```python
from build123d import *

# Parameters (mm, degrees)
BOSS_EXTRUDE1_DEPTH             = 26.5
SKETCH2_W                       = 10
SKETCH2_H                       = 15
BOSS_EXTRUDE2_DEPTH             = 21.1
BOSS_EXTRUDE2_DIRECTION_2_REACH = 46.455
SKETCH3_W                       = 13.25
SKETCH3_H                       = 38
CUT_EXTRUDE1_DEPTH              = 21.1
CUT_EXTRUDE2_DEPTH              = 46.618088518
CUT_EXTRUDE2_DEPTH_BACK         = 46.618088518
SKETCH4_R                       = 1.8
SKETCH5_R                       = 3.5
CUT_EXTRUDE3_DEPTH              = 11.1
SKETCH6_R                       = 1.9
CUT_EXTRUDE4_DEPTH              = 46.618088518
FILLET1_R                       = 5
CHAMFER1_SIZE                   = 0.25


with BuildPart() as part:
    # Sketch1 → Boss-Extrude1 (new body)
    with BuildSketch(Plane.XY):
        Polygon((0, 35), (0, 28), (2.4, 28), (2.4, -10), (7, -10), (7, 35), align=None)
    extrude(amount=BOSS_EXTRUDE1_DEPTH)

    # Sketch2 → Boss-Extrude2 (add)
    with BuildSketch(Plane.XY):
        with Locations((7.4, -2.5)):
            Rectangle(SKETCH2_W, SKETCH2_H)
    extrude(amount=-BOSS_EXTRUDE2_DEPTH)

    # Boss-Extrude2 direction 2: up to this face of the body (flat: up to its plane)
    boss_extrude2_direction_2_end = Plane(part.part.faces().sort_by_distance((4.437265416, 13.926273458, 26.5))[0])
    # Sketch2 → Boss-Extrude2 direction 2 (add, up to the picked face)
    with BuildSketch(Plane.XY, mode=Mode.PRIVATE) as boss_extrude2_direction_2_sk1:
        with Locations((7.4, -2.5)):
            Rectangle(SKETCH2_W, SKETCH2_H)
    boss_extrude2_direction_2_tool1 = split(extrude(boss_extrude2_direction_2_sk1.sketch, amount=BOSS_EXTRUDE2_DIRECTION_2_REACH, mode=Mode.PRIVATE), bisect_by=boss_extrude2_direction_2_end, keep=Keep.BOTH, mode=Mode.PRIVATE)
    add(boss_extrude2_direction_2_tool1.solids().sort_by(Axis((7.4, -2.5, 0), (0, 0, 1)))[0])

    # Sketch3 → Cut-Extrude1 (cut)
    with BuildSketch(Plane(origin=(0, 0, 0), x_dir=(0, 0, -1), z_dir=(1, 0, 0))):
        with Locations((-19.875, 9)):
            Rectangle(SKETCH3_W, SKETCH3_H)
    extrude(amount=CUT_EXTRUDE1_DEPTH, mode=Mode.SUBTRACT)

    # Sketch4 → Cut-Extrude2 (cut, two sides: drawn at the far end of the back side and taken through both)
    with BuildSketch(Plane.XY.offset(-CUT_EXTRUDE2_DEPTH_BACK)):
        with Locations((7.4, -2.5)):
            Circle(SKETCH4_R)
    extrude(amount=CUT_EXTRUDE2_DEPTH + CUT_EXTRUDE2_DEPTH_BACK, mode=Mode.SUBTRACT)

    # Sketch5 → Cut-Extrude3 (cut)
    with BuildSketch(Plane.XY.offset(13.25)):
        with Locations((7.4, -2.5)):
            Circle(SKETCH5_R)
    extrude(amount=-CUT_EXTRUDE3_DEPTH, mode=Mode.SUBTRACT)

    # Sketch6 → Cut-Extrude4 (cut, through all)
    with BuildSketch(Plane(origin=(0, 0, 0), x_dir=(0, 0, -1), z_dir=(1, 0, 0))):
        with Locations(Location((-3, 31.5, 0), (0, 0, 270))):
            Circle(SKETCH6_R)
        with Locations(Location((-23.5, 31.5, 0), (0, 0, 180))):
            Circle(SKETCH6_R)
    extrude(amount=CUT_EXTRUDE4_DEPTH, mode=Mode.SUBTRACT)

    # Fillet1
    fillet1_edges = [part.edges().sort_by_distance(p)[0] for p in [
        (2.4, -10, -3.925),
        (12.4, -10, -3.925),
    ]]
    fillet(fillet1_edges, radius=FILLET1_R - 0.0001)  # a hair under: the kernel refuses the full size

    # Chamfer1
    chamfer1_edges = [part.edges().sort_by_distance(p)[0] for p in [
        (3.864436805, -8.535563195, 13.25),
        (10.935563195, -8.535563195, 13.25),
        (7, 35, 13.25),
        (0, 28, 13.25),
        (0, 35, 13.25),
        (3.5, 28, 26.5),
        (7, 20, 0),
        (4.7, 5, 0),
        (2.4, 5, -10.55),
        (7, 5, 6.625),
        (12.4, 5, -3.925),
        (7, 31.5, 26.5),
        (7, 28, 19.875),
        (2.4, 11.49995, 13.25),
        (9.7, 5, 13.25),
        (7, 16.5, 13.25),
        (3.5, 35, 26.5),
        (2.4, 16.5, 0),
        (1.2, 28, 0),
        (0, 33.4, 3),
        (7, 33.4, 3),
        (0, 31.5, 21.6),
        (7, 31.5, 21.6),
        (0, 31.5, 0),
        (3.5, 35, 0),
        (0, 31.5, 26.5),
        (12.4, -5e-05, 13.25),
    ]]
    chamfer(chamfer1_edges, length=CHAMFER1_SIZE)


solid = part.part
```
Source: CAD feature listing. Evaluate the final solid. Frame: model axes, mm. A direction names the side the tool comes from. Give positions to 0.01 mm unless a question says otherwise; leave off trailing zeros. Write each loop counter-clockwise with the first axis right and the second up, starting at its lowest first coordinate (ties: lowest second). Pieces come first, ordered by that corner, then holes.
1. Material intervals for line 1 along X through (y, z) = (-2.5, -6.25); line 2 along Y through (x, z) = (4, 23.5); line 3 along Y through (x, z) = (7.4, -13.25), sorted ascending.
2. Section query A-A (y = -2.5). Return the cut outline in (x, z), then the cut area to 3 significant figures.
3. Pull-direction query (Z, two-part tool) for faces 1 (the face through (12.4, 0, -4)), 2 (the face through (3, 32, 26.5)), 3 (the face through (3.454, 29.688, 2.429)); classes: +Z half, -Z half, draft (parallel to the pull), parting line (faces both ways), or undercut.
4. First-contact query: pin 1 (3 mm diameter, centred on x = 8.5, z = -4, fed in from +Y); pin 2 (2 mm diameter, centred on y = 7, z = 1.5, fed in from +X); pin 3 (3 mm diameter, centred on x = 3, y = 15, fed in from -Z); pin 4 (2.5 mm diameter, centred on y = 31.5, z = 23.5, fed in from -X). Flat tips, straight axial feed; report the tip coordinate or a pass-through.
5. Section query C-C (y = 31.5). Return the cut outline in (x, z).
6. Access query for faces 4 (the face through (6, 9, 13.25)), 5 (the face through (9, -4, 2.15)), 6 (the face through (4, 20, 0)), 7 (the face through (2.4, 4, 0)). Directions: +Z, -Z, +X, -X, +Y, -Y. A direction counts if a zero-diameter tool reaches every point of the face in a straight line with its end or side. Return the directions, or none.
7. Section query B-B (z = 3). Count the separate pieces of the cut face and the enclosed holes in it, then the cut area to 3 significant figures.
8. Section query D-D (z = 14.5). Return the cut outline in (x, y), then the cut area to 3 significant figures.
Output values:
1. line 1: x = 2.4 to 5.6, 9.2 to 12.4
1. line 2: y = 28 to 29.6, 33.4 to 35
1. line 3: y = -10 to -4.3, -0.7 to 5
2. outline: (2.4, -21.1) - (5.6, -21.1) - (5.6, 2.15) - (3.9, 2.15) - (3.9, 13.25) - (2.65, 13.25) - (2.4, 13) - close; (9.2, -21.1) - (12.4, -21.1) - (12.4, 13) - (12.15, 13.25) - (10.9, 13.25) - (10.9, 2.15) - (9.2, 2.15) - close
2. area: 182 mm2
3. face 1: draft
3. face 2: +Z half
3. face 3: undercut
4. pin 1: stops at y = 5
4. pin 2: stops at x = 7
4. pin 3: stops at z = 0
4. pin 4: passes through
5. outline: (0, 0.25) - (0.25, 0) - (6.75, 0) - (7, 0.25) - (7, 0.85) - (6.75, 1.1) - (0.25, 1.1) - (0, 0.85) - close; (0, 5.15) - (0.25, 4.9) - (6.75, 4.9) - (7, 5.15) - (7, 21.35) - (6.75, 21.6) - (0.25, 21.6) - (0, 21.35) - close; (0, 25.65) - (0.25, 25.4) - (6.75, 25.4) - (7, 25.65) - (7, 26.25) - (6.75, 26.5) - (0.25, 26.5) - (0, 26.25) - close
6. face 4: +Z, +X, -X, -Y
6. face 5: +Z
6. face 6: -Z, +X, -X, +Y
6. face 7: +Z, -Z, -X, -Y
7. separate pieces: 2
7. enclosed holes: 1
7. area: 229 mm2
8. outline: (0, 28.25) - (0.25, 28) - (6.75, 28) - (7, 28.25) - (7, 34.75) - (6.75, 35) - (0.25, 35) - (0, 34.75) - close
8. area: 48.9 mm2
